```python
from build123d import *

# Parameters (mm, degrees)
SKETCH_1_R      = 1.55
EXTRUDE_1_DEPTH = 7
FILLET_1_R      = 4


with BuildPart() as part:
    # Эскиз1 → Бобышка-Вытянуть1 (new body)
    with BuildSketch(Plane.XY):
        with BuildLine():
            Line((18.5, 101.493831222), (124.5, 101.493831222))
            ThreePointArc((124.5, 101.493831222), (130.5, 95.493831222), (124.5, 89.493831222))
            Line((124.5, 89.493831222), (18.5, 89.493831222))
            ThreePointArc((18.5, 89.493831222), (12.5, 95.493831222), (18.5, 101.493831222))
        make_face()
        with Locations((124.5, 95.493831222)):
            Circle(SKETCH_1_R, mode=Mode.SUBTRACT)
        with Locations((18.5, 95.493831222)):
            Circle(SKETCH_1_R, mode=Mode.SUBTRACT)
    extrude(amount=EXTRUDE_1_DEPTH)

    # Эскиз3 → Вырез-Повернуть1 (revolve, cut)
    with BuildSketch(Plane(origin=(0, 95.493831222, 0), x_dir=(1, 0, 0), z_dir=(0, 1, 0))):
        with BuildLine():
            Line((11.788259636, -5.953922017), (11.5, -7.498579905))
            Line((11.5, -7.498579905), (18.5, -7.498579905))
            Line((18.5, -7.498579905), (18.5, -3.65512576))
            Line((18.5, -3.65512576), (18.5, 0.188328385))
            Line((18.5, 0.188328385), (15, 0.188328385))
            Line((15, 0.188328385), (15.100959011, -0.893662386))
            ThreePointArc((15.100959011, -0.893662386), (15.858000965, -0.830944257), (16.616181879, -0.783957185))
            Line((16.616181879, -0.783957185), (17.151991145, -3.65512576))
            Line((17.151991145, -3.65512576), (16.616181879, -6.526294335))
            ThreePointArc((16.616181879, -6.526294335), (14.192702827, -6.320391282), (11.788259636, -5.953922017))
        make_face()
    revolve(axis=Axis((18.5, 95.493831222, 14.092750712), (0, 0, -1)), mode=Mode.SUBTRACT)

    # Эскиз4 → Вырез-Повернуть2 (revolve, cut)
    with BuildSketch(Plane(origin=(0, 95.493831222, 0), x_dir=(1, 0, 0), z_dir=(0, 1, 0))):
        with BuildLine():
            Line((124.5, -6.829517276), (124.5, -8.843780512))
            Line((124.5, -8.843780512), (131.5, -8.843780512))
            Line((131.5, -8.843780512), (131.062493989, -5.564992503))
            ThreePointArc((131.062493989, -5.564992503), (128.910766156, -6.355557055), (126.667936093, -6.829517276))
            Line((126.667936093, -6.829517276), (126.340236608, -4.373648978))
            Line((126.340236608, -4.373648978), (126.825045666, -1.111490634))
            ThreePointArc((126.825045666, -1.111490634), (127.546113951, -1.228496574), (128.261402877, -1.37679228))
            Line((128.261402877, -1.37679228), (128.620585304, 1.040056032))
            Line((128.620585304, 1.040056032), (124.5, 1.040056032))
            Line((124.5, 1.040056032), (124.5, -0.95889034))
            Line((124.5, -0.95889034), (124.5, -4.373648978))
            Line((124.5, -4.373648978), (124.5, -6.829517276))
        make_face()
    revolve(axis=Axis((124.5, 95.493831222, 6.829517276), (0, 0, -1)), mode=Mode.SUBTRACT)

    # Скругление1
    # the kernel refuses this fillet: 4 mm, written as the material it takes off along each edge
    with BuildSketch(Plane(origin=(18.5, 95.493831222, 7), x_dir=(-0.3783138091133085, -0.9256774070021258, 0), z_dir=(-0.9256774070021258, 0.3783138091133085, 0))) as fillet_1_piece_1:
        with BuildLine():
            CenterArc((9.408839679, -4), FILLET_1_R, 90, 42.397861789)
            Line((6.711740364, -1.046077983), (6.657798378, -0.986999543))
            ThreePointArc((6.657798378, -0.986999543), (6.730706082, -0.508362986), (6.828314122, 0.014676005))
            Line((6.828314122, 0.014676005), (6.906956445, 0.08))
            Line((6.906956445, 0.08), (9.408839679, 0.08))
            Line((9.408839679, 0.08), (9.408839679, 0))
        make_face()
    revolve(axis=Axis((18.5, 95.493831222, 7), (0, 0, 1)), revolution_arc=224.458550317, mode=Mode.SUBTRACT)
    with BuildSketch(Plane(origin=(124.5, 95.493831222, 7), x_dir=(0.5555728913657687, -0.8314678360462777, 0), z_dir=(0.8314678360462777, 0.5555728913657687, 0))) as fillet_1_piece_2:
        with BuildLine():
            CenterArc((9.631828356, 4), FILLET_1_R, 219.884952178, 50.115047822)
            Line((9.631828356, 0), (9.631828356, -0.08))
            Line((9.631828356, -0.08), (6.753974623, -0.08))
            Line((6.753974623, -0.08), (6.67467745, -0.010581041))
            ThreePointArc((6.67467745, -0.010581041), (6.578937133, 0.706922708), (6.501107302, 1.383707647))
            Line((6.501107302, 1.383707647), (6.562493989, 1.435007497))
        make_face()
    revolve(axis=Axis((124.5, 95.493831222, 7), (0, 0, -1)), revolution_arc=247.500366369, mode=Mode.SUBTRACT)


solid = part.part
```
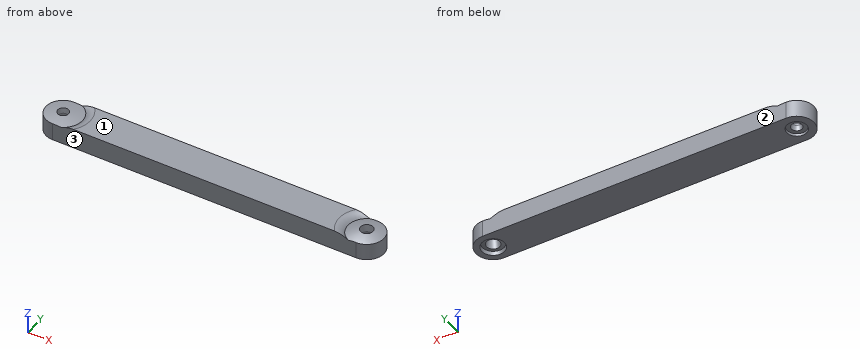
For this review, take the finished solid that the model builds, in its own axes (mm). Face numbers are marked on the shaded views. Coordinates: 2 decimals unless noted, no trailing zeros. Answer as CSV lines item,"result".
Q1. Wall thickness on line 1 along Y through (x, z) = (18.5, 3.1); line 2 along Y through (x, z) = (125, 3.5); line 3 along X through (y, z) = (100.5, 3.25): over which ranges is each line inside the solid? List them lowest first. Write a range as [from, to].
Model answer:
line 1,"y = [89.49, 93.94], [97.04, 101.49]"
line 2,"y = [89.51, 93.59], [97.4, 101.47]"
line 3,"x = [15.19, 127.81]"
Q2. Draft analysis for pull direction Y (two halves, no side actions). For the marked faces 1, 2 and 3, state which applies: released by +Y, released by -Y, zero draft, split by the parting line, or undercut.
Model answer:
face 1,"zero draft"
face 2,"released by +Y"
face 3,"released by -Y"
Q3. Clearance check with flat-ended pins moving along their axes: pin 1 Ø2.5 at (x, y) = (18.5, 95.49) entering from -Z; pin 2 Ø1.5 at (y, z) = (99, 1) entering from -X; pin 3 Ø3 at (y, z) = (100.5, 2) entering from -X. State where each tip first meets the part, or that it passes through.
Model answer:
pin 1,"passes through"
pin 2,"stops at x = 13.17"
pin 3,"stops at x = 13.63"
